Source: CAD feature listing. Evaluate the final solid. Frame: model axes, mm. Coordinates: 2 decimals unless noted, no trailing zeros. Loops run counter-clockwise (first coordinate to the right, second up) from the corner with the lowest first, then second, coordinate; pieces in that order, holes last.
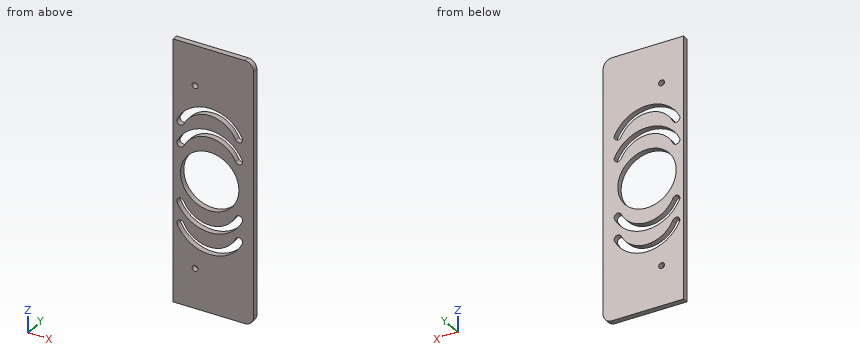
```python
from build123d import *

# Parameters (mm, degrees)
SKETCH1_W           = 139.7
SKETCH1_H           = 457.2
SKETCH1_R           = 50.8
SKETCH1_R_2         = 5.08
BOSS_EXTRUDE1_DEPTH = 9.652
FILLET1_R           = 15.08
CUT_EXTRUDE1_DEPTH  = 9.652


with BuildPart() as part:
    # Sketch1 → Boss-Extrude1 (new body)
    with BuildSketch(Plane(origin=(0, 0, 0), x_dir=(1, 0, 0), z_dir=(0, 1, 0))):
        with Locations((69.85, 228.6)):
            Rectangle(SKETCH1_W, SKETCH1_H)
        with Locations((63.5, 228.6)):
            Circle(SKETCH1_R, mode=Mode.SUBTRACT)
        with Locations((38.1, 69.85)):
            Circle(SKETCH1_R_2, mode=Mode.SUBTRACT)
        with Locations((38.1, 387.35)):
            Circle(SKETCH1_R_2, mode=Mode.SUBTRACT)
    extrude(amount=BOSS_EXTRUDE1_DEPTH)

    # Fillet1
    fillet1_edges = [part.edges().sort_by_distance(p)[0] for p in [
        (139.7, 4.826, -457.2),
        (139.7, 4.826, 0),
    ]]
    fillet(fillet1_edges, radius=FILLET1_R)

    # Sketch3 → Cut-Extrude1 (cut)
    with BuildSketch(Plane.XZ):
        with BuildLine():
            ThreePointArc((18.407865169, -314.71741573), (63.5, -342.9), (108.592134831, -314.71741573))
            ThreePointArc((108.592134831, -314.71741573), (117.08258427, -311.792134831), (120.007865169, -320.28258427))
            ThreePointArc((120.007865169, -320.28258427), (63.5, -355.6), (6.992134831, -320.28258427))
            ThreePointArc((6.992134831, -320.28258427), (9.91741573, -311.792134831), (18.407865169, -314.71741573))
        make_face()
        with BuildLine():
            ThreePointArc((6.992134831, -282.18258427), (63.5, -317.5), (120.007865169, -282.18258427))
            ThreePointArc((120.007865169, -282.18258427), (117.08258427, -273.692134831), (108.592134831, -276.61741573))
            ThreePointArc((108.592134831, -276.61741573), (63.5, -304.8), (18.407865169, -276.61741573))
            ThreePointArc((18.407865169, -276.61741573), (9.91741573, -273.692134831), (6.992134831, -282.18258427))
        make_face()
        with BuildLine():
            ThreePointArc((6.992134831, -136.91741573), (63.5, -101.6), (120.007865169, -136.91741573))
            ThreePointArc((120.007865169, -136.91741573), (117.08258427, -145.407865169), (108.592134831, -142.48258427))
            ThreePointArc((108.592134831, -142.48258427), (63.5, -114.3), (18.407865169, -142.48258427))
            ThreePointArc((18.407865169, -142.48258427), (9.91741573, -145.407865169), (6.992134831, -136.91741573))
        make_face()
        with BuildLine():
            ThreePointArc((6.992134831, -175.01741573), (63.5, -139.7), (120.007865169, -175.01741573))
            ThreePointArc((120.007865169, -175.01741573), (117.08258427, -183.507865169), (108.592134831, -180.58258427))
            ThreePointArc((108.592134831, -180.58258427), (63.5, -152.4), (18.407865169, -180.58258427))
            ThreePointArc((18.407865169, -180.58258427), (9.91741573, -183.507865169), (6.992134831, -175.01741573))
        make_face()
    extrude(amount=-CUT_EXTRUDE1_DEPTH, mode=Mode.SUBTRACT)


solid = part.part
```
Q1. First-contact query: pin 1 Ø10 at (x, z) = (54, -368) entering from -Y; pin 2 Ø9 at (x, z) = (38.1, -69.85) entering from +Y. Flat tips, straight axial feed; report the tip coordinate or a pass-through.
Q2. Section query C-C on x = 83.5. Return the cut outline in (y, z).
Q3. Material intervals for line 1 along Z through (x, y) = (63.5, 7.5); line 2 along X through (y, z) = (3.75, -387.35); line 3 along Z through (x, y) = (72, 4.75), sorted ascending.
Q4. Section query D-D on z = -120. Return the cut outline in (x, y), then the cut area to 3 significant figures.
Q5. Section query B-B on y = 3. Return the cut outline in (x, z) (3 decimals).
Q6. Section query A-A on z = -228.6. Return the cut outline in (x, y), then the cut area to 3 significant figures.
Resolved:
1. pin 1: stops at y = 0
1. pin 2: passes through
2. outline: (0, -457.2) - (9.65, -457.2) - (9.65, -352.33) - (0, -352.33) - close; (0, -338.74) - (9.65, -338.74) - (9.65, -314.23) - (0, -314.23) - close; (0, -300.64) - (9.65, -300.64) - (9.65, -275.3) - (0, -275.3) - close; (0, -181.9) - (9.65, -181.9) - (9.65, -156.56) - (0, -156.56) - close; (0, -142.97) - (9.65, -142.97) - (9.65, -118.46) - (0, -118.46) - close; (0, -104.87) - (9.65, -104.87) - (9.65, 0) - (0, 0) - close
3. line 1: z = -457.2 to -355.6, -342.9 to -317.5, -304.8 to -279.4, -177.8 to -152.4, -139.7 to -114.3, -101.6 to 0
3. line 2: x = 0 to 33.02, 43.18 to 139.7
3. line 3: z = -457.2 to -355.02, -342.17 to -316.92, -304.07 to -278.68, -178.52 to -153.13, -140.28 to -115.03, -102.18 to 0
4. outline: (0, 0) - (19.06, 0) - (19.06, 9.65) - (0, 9.65) - close; (40.28, 0) - (86.72, 0) - (86.72, 9.65) - (40.28, 9.65) - close; (107.94, 0) - (139.7, 0) - (139.7, 9.65) - (107.94, 9.65) - close
4. area: 939 mm2
5. outline: (0, -457.2) - (124.62, -457.2) arc R15.08 ccw to (139.7, -442.12) - (139.7, -15.08) arc R15.08 ccw to (124.62, 0) - (0, 0) - close; hole (6.992, -320.283) arc R62.865 ccw to (120.008, -320.283) arc R6.35 ccw to (108.592, -314.717) arc R50.165 cw to (18.408, -314.717) arc R6.35 ccw to start; hole (6.992, -282.183) arc R62.865 ccw to (120.008, -282.183) arc R6.35 ccw to (108.592, -276.617) arc R50.165 cw to (18.408, -276.617) arc R6.35 ccw to start; hole (6.992, -175.017) arc R6.35 ccw to (18.408, -180.583) arc R50.165 cw to (108.592, -180.583) arc R6.35 ccw to (120.008, -175.017) arc R62.865 ccw to start; hole (6.992, -136.917) arc R6.35 ccw to (18.408, -142.483) arc R50.165 cw to (108.592, -142.483) arc R6.35 ccw to (120.008, -136.917) arc R62.865 ccw to start; hole circle Ø101.6 at (63.5, -228.6); hole circle Ø10.16 at (38.1, -387.35); hole circle Ø10.16 at (38.1, -69.85)
6. outline: (0, 0) - (12.7, 0) - (12.7, 9.65) - (0, 9.65) - close; (114.3, 0) - (139.7, 0) - (139.7, 9.65) - (114.3, 9.65) - close
6. area: 368 mm2
